from build123d import *

# Parameters (mm, degrees)
FURO_DE_DI_METRO_5_5_5_5_1_REACH  = 126.138
FURO_DE_DI_METRO_5_5_5_5_1_BORE_R = 2.75


with BuildPart() as part:
    # Esboço1 → Revolução1 (revolve)
    with BuildSketch(Plane.XY, mode=Mode.PRIVATE) as revolu_o1_sk:
        Polygon((0, 3.5), (0, 7.5), (108.5, 7.5), (108.5, 6), (123, 6), (123, 4.5), (100, 4.5), (100, 4), (11, 4), (11, 3.5), align=None)
    revolve(revolu_o1_sk.sketch.rotate(Axis((123, 0, 0), (-1, 0, 0)), 90), axis=Axis((123, 0, 0), (-1, 0, 0)))

    # Furo de diâmetro Ø5.5 (5.5)1 bore → Furo de diâmetro Ø5.5 (5.5)1 (cut, up to next)
    with BuildSketch(Plane(origin=(0, 0, -7.5), x_dir=(-1, 0, 0), z_dir=(0, 0, -1)), mode=Mode.PRIVATE) as furo_de_di_metro_5_5_5_5_1_sk1:
        with Locations((-8, 0)):
            Circle(FURO_DE_DI_METRO_5_5_5_5_1_BORE_R)
    furo_de_di_metro_5_5_5_5_1_tool1 = extrude(furo_de_di_metro_5_5_5_5_1_sk1.sketch, amount=-FURO_DE_DI_METRO_5_5_5_5_1_REACH, mode=Mode.PRIVATE) & part.part
    furo_de_di_metro_5_5_5_5_1 = furo_de_di_metro_5_5_5_5_1_tool1.solids().sort_by_distance((8, 0, -7.5))[0]
    add(furo_de_di_metro_5_5_5_5_1, mode=Mode.SUBTRACT)

    # Espelhar1: Furo de diâmetro Ø5.5 (5.5)1 across plane
    add(furo_de_di_metro_5_5_5_5_1.mirror(Plane.XY), mode=Mode.SUBTRACT)


solid = part.part
Source: CAD feature listing. Evaluate the final solid. Frame: model axes, mm. A direction names the side the tool comes from. Round coordinates to 2 decimals unless told otherwise and drop trailing zeros. Loops run counter-clockwise (first coordinate to the right, second up) from the corner with the lowest first, then second, coordinate; pieces in that order, holes last.
Q1. Section A-A, the plane z = 0. Return loops of the section in (x, y), plus the area to 4 significant figures.
Q2. Section C-C, the plane x = 8. Return loops of the section in (y, z).
Q3. Mould query, pull axis X, two halves, no side actions, for faces 1 (the face through (100, 3, 3)), 2 (the face through (115.852, -1.802, -5.723)), 3 (the face through (10.747, 0.121, -4.87)). Classes: pulls with the +X half, pulls with the -X half, needs draft (parallel to the pull), parting line crosses it, or undercut.
Q4. Section B-B, the plane y = 0. Return loops of the section in (x, z), plus the area to 4 significant figures.
Q5. Access query for faces 4 (the face through (0, -1.8, 3.2)), 5 (the face through (108.5, -6, -2)). Directions: +Z, -Z, +X, -X, +Y, -Y. A direction counts if a zero-diameter tool reaches every point of the face in a straight line with its end or side. Return the directions, or none.
Q6. First-contact query: P1, Ø6, axis at y = 0, z = 4, coming from the -X side; P2, Ø3, axis at x = 75, y = 4, coming from the -Z side; P3, Ø2, axis at x = 20.5, y = -4.5, coming from the +Z side; P4, Ø1.5, axis at x = 65, y = -2, coming from the -Z side. Flat tips, straight axial feed; report the tip coordinate or a pass-through.
Q7. Ray query, line 1 (Y direction, x = 109, z = 0); line 2 (Y direction, x = 42, z = 0); line 3 (X direction, y = 6.75, z = -2.5). Return the intervals inside material, ascending.
Q8. Section D-D, the plane x = 60.5. Return loops of the section in (y, z).
Solutions:
1. outline: (0, -7.5) - (108.5, -7.5) - (108.5, -6) - (123, -6) - (123, -4.5) - (100, -4.5) - (100, -4) - (11, -4) - (11, -3.5) - (0, -3.5) - close; (0, 3.5) - (11, 3.5) - (11, 4) - (100, 4) - (100, 4.5) - (123, 4.5) - (123, 6) - (108.5, 6) - (108.5, 7.5) - (0, 7.5) - close
1. area: 805.5 mm2
2. outline: (-2.75, -6.98) - (-2.75, -2.17) arc R3.5 cw to (-2.75, 2.17) - (-2.75, 6.98) arc R7.5 ccw to start; (2.75, -6.98) arc R7.5 ccw to (2.75, 6.98) - (2.75, 2.17) arc R3.5 cw to (2.75, -2.17) - close
3. face 1: pulls with the +X half
3. face 2: needs draft
3. face 3: undercut
4. outline: (0, -7.5) - (5.25, -7.5) - (5.25, -3.5) - (0, -3.5) - close; (0, 3.5) - (5.25, 3.5) - (5.25, 7.5) - (0, 7.5) - close; (10.75, -7.5) - (108.5, -7.5) - (108.5, -6) - (123, -6) - (123, -4.5) - (100, -4.5) - (100, -4) - (11, -4) - (11, -3.5) - (10.75, -3.5) - close; (10.75, 3.5) - (11, 3.5) - (11, 4) - (100, 4) - (100, 4.5) - (123, 4.5) - (123, 6) - (108.5, 6) - (108.5, 7.5) - (10.75, 7.5) - close
4. area: 761.5 mm2
5. face 4: +Z, -Z, -X, +Y, -Y
5. face 5: +X
6. P1: stops at x = 0
6. P2: stops at z = -7.07
6. P3: stops at z = 6.63
6. P4: stops at z = -7.4
7. line 1: y = -6 to -4.5, 4.5 to 6
7. line 2: y = -7.5 to -4, 4 to 7.5
7. line 3: x = 0 to 108.5
8. outline: circle Ø15 at (0, 0); hole circle Ø8 at (0, 0)
